```python
from build123d import *

# Parameters (mm, degrees)
ESQUISSE1_W      = 79
ESQUISSE1_H      = 145
EXTRUSION1_DEPTH = 5
EXTRUSION2_REACH = 110.909


with BuildPart() as part:
    # Esquisse1 → Extrusion1 (new body)
    with BuildSketch(Plane(origin=(0, 0, 0), x_dir=(1, 0, 0), z_dir=(0, 1, 0))):
        with Locations((-4.262748952, -27.104127358)):
            Rectangle(ESQUISSE1_W, ESQUISSE1_H)
    extrude(amount=EXTRUSION1_DEPTH)

    # Esquisse2 → Extrusion2 (cut, up to next)
    with BuildSketch(Plane(origin=(0, 5, 0), x_dir=(1, 0, 0), z_dir=(0, 1, 0)), mode=Mode.PRIVATE) as extrusion2_sk1:
        Polygon((-16.762748952, -22.604127358), (-11.762748952, -22.604127358), (-11.762748952, -31.604127358), (3.237251048, -31.604127358), (3.237251048, -22.604127358), (8.237251048, -22.604127358), (8.237251048, -94.604127358), (3.237251048, -94.604127358), (3.237251048, -85.604127358), (-11.762748952, -85.604127358), (-11.762748952, -94.604127358), (-16.762748952, -94.604127358), align=None)
    extrusion2_tool1 = extrude(extrusion2_sk1.sketch, amount=-EXTRUSION2_REACH, mode=Mode.PRIVATE) & part.part
    add(extrusion2_tool1.solids().sort_by_distance((-4.262749, 5, 58.604127))[0], mode=Mode.SUBTRACT)


solid = part.part
```
For this review, take the finished solid that the model builds, in its own axes (mm). A direction names the side the tool comes from. Give positions to 0.01 mm unless a question says otherwise; leave off trailing zeros. Write each loop counter-clockwise with the first axis right and the second up, starting at its lowest first coordinate (ties: lowest second). Pieces come first, ordered by that corner, then holes.
Item 1: The part is to be moulded in two halves that separate along Z. For faces 1 (the face through (-4, 3, 31.604)), 2 (the face through (-5, 2, -45.396)), 3 (the face through (-43.763, 2, 28)), say which applies: +Z half, -Z half, draft (parallel to the pull), parting line (faces both ways), or undercut.
Item 2: Take a section at B-B (y = 2.75). Give the boundary of the cut face in (x, z).
Item 3: Machinability: for faces 4 (the face through (6, 3, 94.604)), 5 (the face through (-5, 2, 99.604)), which of the approach directions +Z, -Z, +X, -X, +Y, -Y give a long, thin tool a straight path to every point of the face, cutting with its end or side? Answer none if there is none.
Item 4: Take a section at C-C (x = 5.5). Give the boundary of the cut face in (y, z), and give its area (3 significant figures).
Item 5: Take a section at A-A (z = 38). Give the boundary of the cut face in (x, y).
Item 6: Wall thickness on probe 1 along X at (y, z) = (3.95, 91); probe 2 along X at (y, z) = (2.9, 58); probe 3 along Z at (x, y) = (-13.5, 1.95): over which ranges is each line inside the solid? List them lowest first.
Established:
1. face 1: undercut
1. face 2: -Z half
1. face 3: draft
2. outline: (-43.76, -45.4) - (35.24, -45.4) - (35.24, 99.6) - (-43.76, 99.6) - close; hole (-16.76, 22.6) - (-11.76, 22.6) - (-11.76, 31.6) - (3.24, 31.6) - (3.24, 22.6) - (8.24, 22.6) - (8.24, 94.6) - (3.24, 94.6) - (3.24, 85.6) - (-11.76, 85.6) - (-11.76, 94.6) - (-16.76, 94.6) - close
3. face 4: +Y, -Y
3. face 5: +Z, +X, -X, +Y, -Y
4. outline: (0, -45.4) - (5, -45.4) - (5, 22.6) - (0, 22.6) - close; (0, 94.6) - (5, 94.6) - (5, 99.6) - (0, 99.6) - close
4. area: 365 mm2
5. outline: (-43.76, 0) - (-16.76, 0) - (-16.76, 5) - (-43.76, 5) - close; (8.24, 0) - (35.24, 0) - (35.24, 5) - (8.24, 5) - close
6. probe 1: x = -43.76 to -16.76, -11.76 to 3.24, 8.24 to 35.24
6. probe 2: x = -43.76 to -16.76, 8.24 to 35.24
6. probe 3: z = -45.4 to 22.6, 94.6 to 99.6
